Answer from the drawing. Dimensions are ordinates in mm from the lowest x, y and z of the part. Give positions to 0.01 mm unless a question says otherwise; leave off trailing zeros. Write each loop counter-clockwise with the first axis right and the second up, starting at its lowest first coordinate (ties: lowest second). Pieces come first, ordered by that corner, then holes. Notation, with made-up numbers: (86, 42.5) -> (91, 42.5) arc R23 ccw to (91, 74.5) -> close; hole circle Ø10 at (7.25, 9). An arc over 180 degrees is marked (long way). Write item = value, one per line.
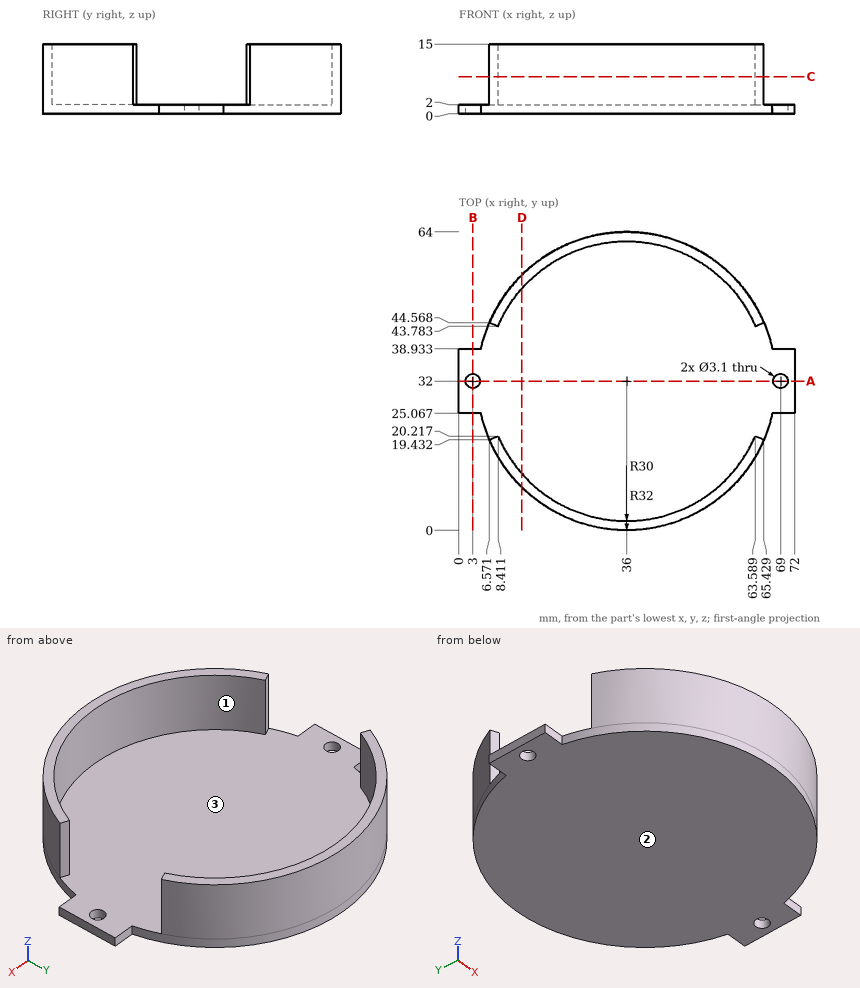
(1) The part is cut by section A-A on y = 32. Determine the outline of the cut face in (x, z).
Checks:
outline = (0, 0) -> (1.45, 0) -> (1.45, 2) -> (0, 2) -> close; (4.55, 0) -> (67.45, 0) -> (67.45, 2) -> (4.55, 2) -> close; (70.55, 0) -> (72, 0) -> (72, 2) -> (70.55, 2) -> close
(2) The part is cut by section C-C on z = 8. Determine the outline of the cut face in (x, y).
Checks:
outline = (6.57, 19.43) arc R32 ccw to (65.43, 19.43) -> (63.59, 20.22) arc R30 cw to (8.41, 20.22) -> close; (6.57, 44.57) -> (8.41, 43.78) arc R30 cw to (63.59, 43.78) -> (65.43, 44.57) arc R32 ccw to start
(3) For a pull along X with two mould halves and no side action, classify the marked faces 1, 2 and 3 as released by +X, released by -X, zero draft, split by the parting line, or undercut.
Checks:
face_1 = undercut
face_2 = zero draft
face_3 = undercut
(4) Consider L1, parallel to Y at x = 3, z = 1; L2, parallel to Z at x = 65.5, y = 44; L3, parallel to Y at x = 32, z = 3.75. Determine where each line is inside the solid, lowest interval first.
Checks:
L1 = 25.07 to 30.45, 33.55 to 38.93
L2 = 0 to 2
L3 = 0.25 to 2.27, 61.73 to 63.75
(5) Given P1, Ø6, axis at x = 36.5, y = 32, coming from the -Z side; P2, Ø8, axis at y = 55.5, z = 3.5, coming from the +X side; P3, Ø3, axis at x = 3, y = 32, coming from the -Z side; P4, Ø3, axis at x = 59.5, z = 3, coming from the -Y side, each flat-ended and moving along its own axis, determine where each tip first touches the part or whether it passes through.
Checks:
P1 = 0
P2 = 61.37
P3 = through
P4 = 8.76
(6) The part is cut by section D-D on x = 13.5. Determine the outline of the cut face in (y, z).
Checks:
outline = (9.25, 0) -> (54.75, 0) -> (54.75, 15) -> (51.84, 15) -> (51.84, 2) -> (12.16, 2) -> (12.16, 15) -> (9.25, 15) -> close
(7) The part is cut by section B-B on x = 3. Determine the outline of the cut face in (y, z).
Checks:
outline = (25.07, 0) -> (30.45, 0) -> (30.45, 2) -> (25.07, 2) -> close; (33.55, 0) -> (38.93, 0) -> (38.93, 2) -> (33.55, 2) -> close
